from build123d import *

# Parameters (mm, degrees)
EXTRUDE_1_DEPTH     = 43
CUT_EXTRUDE_1_REACH = 45
SKETCH_2_R          = 3


with BuildPart() as part:
    # 草图1 → 凸台-拉伸1 (new body)
    with BuildSketch(Plane.XY):
        Polygon((4.090282793, -2.145441681), (3.903148395, 2.469567967), (-0.187134399, 4.615009648), (-4.090282793, 2.145441681), (-3.903148395, -2.469567967), (0.187134399, -4.615009648), align=None)
    extrude(amount=EXTRUDE_1_DEPTH)

    # 草图2 → 切除-拉伸1 (cut, up to next)
    with BuildSketch(Plane.XY.offset(43), mode=Mode.PRIVATE) as cut_extrude_1_sk1:
        Circle(SKETCH_2_R)
    cut_extrude_1_tool1 = extrude(cut_extrude_1_sk1.sketch, amount=-CUT_EXTRUDE_1_REACH, mode=Mode.PRIVATE) & part.part
    add(cut_extrude_1_tool1.solids().sort_by_distance((0, 0, 43))[0], mode=Mode.SUBTRACT)


solid = part.part
Read the model definition and answer for the solid it produces. Units are mm, in the model's axes. Coordinates: 2 decimals unless noted, no trailing zeros. Loops run counter-clockwise (first coordinate to the right, second up) from the corner with the lowest first, then second, coordinate; pieces in that order, holes last. Notation, with made-up numbers: (-4, 46.5) - (32, 46.5) arc R26 ccw to (32, 65.5) - close; hole circle Ø1 at (59, 64). An arc over 180 degrees is marked (long way). Answer in a Markdown table with one row per item.
Q1. Given P1, Ø2, axis at y = 3.5, z = 8.5, coming from the -X side; P2, Ø1, axis at y = 1, z = 14, coming from the +X side; P3, Ø1.5, axis at y = -3.5, z = 10, coming from the -X side, each flat-ended and moving along its own axis, determine where each tip first touches the part or whether it passes through.
Here are the results:
| item | result |
|---|---|
| P1 | stops at x = -3.53 |
| P2 | stops at x = 3.98 |
| P3 | stops at x = -3.37 |
Q2. Find section D-D on x = 3.5. Write down the section's boundary in (y, z).
Here are the results:
| item | result |
|---|---|
| outline | (-2.52, 0) - (2.68, 0) - (2.68, 43) - (-2.52, 43) - close |
Q3. Find section C-C on y = 0. Write down the section's boundary in (x, z), plus the area to 3 significant figures.
Here are the results:
| item | result |
|---|---|
| outline | (-4, 0) - (-3, 0) - (-3, 43) - (-4, 43) - close; (3, 0) - (4, 0) - (4, 43) - (3, 43) - close |
| area | 86.3 mm^2 |
Q4. Find section B-B on z = 16. Write down the section's boundary in (x, y) (3 decimals), plus the area to 3 significant figures.
Here are the results:
| item | result |
|---|---|
| outline | (-4.09, 2.145) - (-3.903, -2.47) - (0.187, -4.615) - (4.09, -2.145) - (3.903, 2.47) - (-0.187, 4.615) - close; hole circle Ø6 at (0, 0) |
| area | 27.2 mm^2 |
Q5. Find section A-A on x = -1. Write down the section's boundary in (y, z), plus the area to 3 significant figures.
Here are the results:
| item | result |
|---|---|
| outline | (-3.99, 0) - (-2.83, 0) - (-2.83, 43) - (-3.99, 43) - close; (2.83, 0) - (4.1, 0) - (4.1, 43) - (2.83, 43) - close |
| area | 105 mm^2 |
Q6. Straight lines are drawn through the part: line 1 along X through (y, z) = (-0.75, 6.5); line 2 along Y through (x, z) = (0, 33); line 3 along Y through (x, z) = (2.5, 27). For each, find the intervals that lie inside material, in ascending order. Write a range as [from, to].
Here are the results:
| item | result |
|---|---|
| line 1 | x = [-3.97, -2.9], [2.9, 4.03] |
| line 2 | y = [-4.52, -3], [3, 4.52] |
| line 3 | y = [-3.15, -1.66], [1.66, 3.21] |
Q7. The mould has two halves that part along X. Classify faces 1 (the cylindrical face through (-3, 0, 22)), 2 (the flat face through (1, -3, 0)), 3 (the flat face through (2.11, -3.4, 21.2)): pulls with the +X half, pulls with the -X half, needs draft (parallel to the pull), parting line crosses it, or undercut.
Here are the results:
| item | result |
|---|---|
| face 1 | undercut |
| face 2 | needs draft |
| face 3 | pulls with the +X half |
